```python
from build123d import *

# Parameters (mm, degrees)
SKETCH_8_W          = 15
SKETCH_8_H          = 15
EXTRUDE_3_DEPTH     = 3
SKETCH_9_W          = 12
SKETCH_9_H          = 12
EXTRUDE_4_DEPTH     = 15
SKETCH_10_R         = 1.6
CUT_EXTRUDE_2_DEPTH = 24.717082451
FILLET_2_R          = 3


with BuildPart() as part:
    # ｽｹｯﾁ8 → ﾎﾞｽ - 押し出し3 (new body)
    with BuildSketch(Plane.XY):
        Rectangle(SKETCH_8_W, SKETCH_8_H)
    extrude(amount=EXTRUDE_3_DEPTH)

    # ｽｹｯﾁ9 → ﾎﾞｽ - 押し出し4 (add)
    with BuildSketch(Plane.XY.offset(3)):
        Rectangle(SKETCH_9_W, SKETCH_9_H)
    extrude(amount=EXTRUDE_4_DEPTH)

    # ｽｹｯﾁ10 → ｶｯﾄ - 押し出し2 (cut, through all)
    with BuildSketch(Plane.ZY.offset(6)):
        with Locations((10.5, 0)):
            Circle(SKETCH_10_R)
    extrude(amount=-CUT_EXTRUDE_2_DEPTH, mode=Mode.SUBTRACT)

    # ﾌｨﾚｯﾄ2
    fillet_2_edges = [part.edges().sort_by_distance(p)[0] for p in [
        (0, 7.5, 0),
        (-7.5, 0, 0),
        (0, -7.5, 0),
        (7.5, 0, 0),
    ]]
    fillet(fillet_2_edges, radius=FILLET_2_R - 0.0001)  # a hair under: the kernel refuses the full size


solid = part.part
```
Can you work these out from the model? Positions are in its coordinate system, mm. A direction names the side the tool comes from. Coordinates: 2 decimals unless noted, no trailing zeros. Loops run counter-clockwise (first coordinate to the right, second up) from the corner with the lowest first, then second, coordinate; pieces in that order, holes last. Notation, with made-up numbers: (-11, 75.25) -> (38, 75.25) arc R9 ccw to (38, 79.25) -> close; hole circle Ø5 at (-24.75, 12). An arc over 180 degrees is marked (long way). Put each result on its own line as item: value. Start each with the question number.
Q1. I want a section at B-B (z = 10.5). Write out the boundary of the cut face in (x, y), plus the area to 3 significant figures.
Q2. Thinking about a two-plate mould opening in Z: for faces 1 (the face through (0.11, -6.64, 0.9)), 2 (the face through (0, 0, 18)), 3 (the face through (-0.08, 0.07, 8.9)), which applies, pulls with the +Z half, pulls with the -Z half, needs draft (parallel to the pull), parting line crosses it, or undercut?
Q3. I want a section at D-D (z = 7.5). Write out the boundary of the cut face in (x, y), plus the area to 3 significant figures.
Q4. For faces 4 (the face through (0, -6, 10)), 5 (the face through (6, -0.1, 8.7)), 6 (the face through (0, 6, 10)), which set-ups out of +Z, -Z, +X, -X, +Y, -Y let a thin tool reach every point of the face, with its end or its side?
Q5. If I drill on line 1 (Y direction, x = -0.25, z = 10.5); line 2 (X direction, y = -0.75, z = 8.5); line 3 (Y direction, x = -2.25, z = 10), over which ranges is the centre line in solid material (lowest first)? Write a range as [from, to].
Q6. I'm going to push flat-ended pins straight in: P1, Ø3.5, axis at x = 0.5, z = 11.5, coming from the +Y side; P2, Ø5, axis at y = 3.5, z = 9.5, coming from the +X side. Where does each tip first touch, or does it pass through?
Taken from the geometry:
1. outline: (-6, -6) -> (6, -6) -> (6, -1.6) -> (-6, -1.6) -> close; (-6, 1.6) -> (6, 1.6) -> (6, 6) -> (-6, 6) -> close
1. area: 106 mm2
2. face 1: pulls with the -Z half
2. face 2: pulls with the +Z half
2. face 3: undercut
3. outline: (-6, -6) -> (6, -6) -> (6, 6) -> (-6, 6) -> close
3. area: 144 mm2
4. face 4: +Z, +X, -X, -Y
4. face 5: +Z, +X, +Y, -Y
4. face 6: +Z, +X, -X, +Y
5. line 1: y = [-6, -1.6], [1.6, 6]
5. line 2: x = [-6, 6]
5. line 3: y = [-6, -1.52], [1.52, 6]
6. P1: stops at y = 6
6. P2: stops at x = 6
